Autodesk Inventor part; units mm, degrees
ref_plane "Work Plane1" through (0, 0, -16.51) normal (0, 0, 1) x (1, 0, 0)
ref_plane "Work Plane2" through (0, 0, -22.86) normal (0, 0, 1) x (1, 0, 0)
ref_plane "YZ Plane" through (0, 0, 0) normal (1, 0, 0) x (0, 1, 0)
sketch "Sketch1" plane through (0, 0, 0) normal (0, 1, 0) x (-1, 0, 0)
  line L0 (0, 0) -> (-48.9966, 0)
  line L1 (-48.9966, 0) -> (-48.9966, -45.72)
  line L2 (-48.9966, -45.72) -> (0, -45.72)
  line L3 (0, -45.72) -> (0, 0)
  dimension "d0" = 48.9966
  dimension "d1" = 45.72
extrude "Extrusion1" add sketch "Sketch1" along normal blind 6.35
sketch "Sketch3" plane through (0, 6.35, 0) normal (0, 1, 0) x (1, 0, 0)
  line L0 (0, 45.72) -> (0, 0)
  line L1 (48.9966, 0) -> (48.9966, 45.72)
  line L2 (0, 29.21) -> (48.9966, 29.21)
  line L3 (48.9966, 29.21) -> (48.9966, 16.51)
  line L4 (48.9966, 16.51) -> (0, 16.51)
  line L5 (0, 16.51) -> (0, 29.21)
  line L6 (48.9966, 45.72) -> (0, 45.72)
  dimension "d4" = 12.7
  dimension "d5" = 16.51
sketch "Sketch4" plane through (0, 6.35, 0) normal (0, 1, 0) x (1, 0, 0)
  circle A0 centre (6.35, 39.37) radius 2.1364
  circle A1 centre (42.6466, 39.37) radius 3.0733
  line L0 (48.9966, 45.72) -> (0, 45.72)
  line L1 (48.9966, 0) -> (48.9966, 45.72)
  line L2 (0, 45.72) -> (0, 0)
  circle A2 centre (6.35, 6.35) radius 2.2799
  circle A3 centre (42.6466, 6.35) radius 1.194
  line L3 (0, 0) -> (48.9966, 0)
  dimension "d6" = 6.1465
  dimension "d7" = 6.35
  dimension "d8" = 6.35
  dimension "d9" = 6.35
  dimension "d10" = 6.35
  dimension "d11" = 6.35
  dimension "d12" = 6.35
  dimension "d13" = 6.35
  dimension "d14" = 6.35
hole "Hole1" at (6.35, 6.35, -39.37) at (42.6466, 6.35, -39.37) at (42.6466, 6.35, -6.35) at (6.35, 6.35, -6.35) direction (0, -1, 0) diameter 3.4 depth 10 tip angle 118
fillet "Fillet1" radius 0.2 4 edges at (42.6466, 6.35, -41.07) (6.35, 6.35, -41.07) (42.6466, 6.35, -8.05) (6.35, 6.35, -8.05)
ref_plane "Work Plane1" through (0, 0, -16.51) normal (0, 0, 1) x (1, 0, 0)
sketch "Sketch5" plane through (0, 0, -16.51) normal (0, 0, 1) x (1, 0, 0)
  line L0 (0, 6.35) -> (48.9966, 6.35)
  line L1 (48.9966, 6.35) -> (0, 6.35)
  arc A0 (48.9966, 6.35) -> (0, 6.35) centre (24.4983, 6.35) ccw
  point P0 (0, 0)
extrude "Extrusion2" add sketch "Sketch5" along normal blind 5.08
ref_plane "Work Plane2" through (0, 0, -22.86) normal (0, 0, 1) x (1, 0, 0)
mirror "Mirror1" about plane through (0, 0, -22.86) normal (0, 0, 1) of "Extrusion2"
sketch "Sketch6" plane through (0, 0, -11.43) normal (0, 0, 1) x (1, 0, 0)
  circle A0 centre (24.4983, 17.78) radius 3.175
  line L0 (0, 6.35) -> (48.9966, 6.35)
  point P0 (0, 0)
  point P1 (24.4983, 6.35)
  point P2 (24.4983, 6.35)
  dimension "d27" = 11.43
  dimension "d28" = 6.35
extrude "Extrusion3" cut sketch "Sketch6" against normal up to surface (5.08 mm away)
sketch "Sketch8" plane through (24.4983, 6.35, -29.21) normal (0, 0, 1) x (1, 0, 0)
  circle A0 centre (0, 11.43) radius 3.175
  circle A1 centre (0, 11.43) radius 5.08
  point P0 (-24.4983, -6.35)
  dimension "d34" = 10.16
extrude "Extrusion5" cut sketch "Sketch8" against normal blind 25.4 contours A0 | A1
properties part number "Carriage Top" material "Aluminum 6061"
Here's how the part is built. I have some questions about the finished solid (model axes, mm). A direction names the side the tool comes from. Coordinates: 2 decimals unless noted, no trailing zeros. Loops run counter-clockwise (first coordinate to the right, second up) from the corner with the lowest first, then second, coordinate; pieces in that order, holes last. Notation, with made-up numbers: (64.5, 31) -> (107.5, 31) arc R23 ccw to (107.5, 53) -> close; hole circle Ø6 at (42, 21.25). An arc over 180 degrees is marked (long way). Return JSON: item names as keys, results as strings.
1) Thinking about a two-plate mould opening in Z: for faces 5 (the face through (0, 3, -23)), 6 (the face through (30, 16, -34.29)), 7 (the face through (30, 16, -29.21)), which applies, +Z half, -Z half, draft (parallel to the pull), parting line (faces both ways), or undercut?
Results below:
{"face 5": "draft", "face 6": "-Z half", "face 7": "undercut"}
2) I need wall thicknesses on line 1 (X direction, y = 1.5, z = -39.37); line 2 (Z direction, x = 6.35, y = 5.25); line 3 (Z direction, x = 6.5, y = 21.5). Which ranges of each line are inside material? Lowest first, please. Write a range as from..to.
Results below:
{"line 1": "0..4.65, 8.05..40.95, 44.35..49", "line 2": "-45.72..-41.07, -37.67..-8.05, -4.65..0", "line 3": "-34.29..-29.21, -16.51..-11.43"}
3) For faces 1 (the face through (23.837, 22.817, -31.714)), 2 (the face through (4.917, 3.032, -5.436)), 3 (the face through (25, 6.35, -6)), 4 (the face through (25, 6.35, -23)), which set-ups out of +Z, -Z, +X, -X, +Y, -Y let a thin tool reach every point of the face, with its end or its side?
Results below:
{"face 1": "-Z", "face 2": "+Y, -Y", "face 3": "+Z, +X, -X, +Y", "face 4": "+X, -X, +Y"}
4) If we section it at A-A, the plane z = -39.37: Write out the boundary of the cut face in (x, y), then the cut area to 3 significant figures.
Results below:
{"outline": "(0, 0) -> (4.65, 0) -> (4.65, 6.15) arc R0.2 ccw to (4.45, 6.35) -> (0, 6.35) -> close; (8.05, 0) -> (40.95, 0) -> (40.95, 6.15) arc R0.2 ccw to (40.75, 6.35) -> (8.25, 6.35) arc R0.2 ccw to (8.05, 6.15) -> close; (44.35, 0) -> (49, 0) -> (49, 6.35) -> (44.55, 6.35) arc R0.2 ccw to (44.35, 6.15) -> close", "area": "268 mm²"}
5) If we section it at B-B, the plane x = 6.35: Write out the boundary of the cut face in (y, z), then the cut area to 3 significant figures.
Results below:
{"outline": "(0, -45.72) -> (6.35, -45.72) -> (6.35, -41.27) arc R0.2 ccw to (6.15, -41.07) -> (0, -41.07) -> close; (0, -37.67) -> (6.15, -37.67) arc R0.2 ccw to (6.35, -37.47) -> (6.35, -34.29) -> (22.81, -34.29) -> (22.81, -29.21) -> (6.35, -29.21) -> (6.35, -16.51) -> (22.81, -16.51) -> (22.81, -11.43) -> (6.35, -11.43) -> (6.35, -8.25) arc R0.2 ccw to (6.15, -8.05) -> (0, -8.05) -> close; (0, -4.65) -> (6.15, -4.65) arc R0.2 ccw to (6.35, -4.45) -> (6.35, 0) -> (0, 0) -> close", "area": "414 mm²"}
6) If we section it at C-C, the plane y = 7: Write out the boundary of the cut face in (x, z).
Results below:
{"outline": "(0.01, -34.29) -> (48.99, -34.29) -> (48.99, -29.21) -> (0.01, -29.21) -> close; (0.01, -16.51) -> (48.99, -16.51) -> (48.99, -11.43) -> (0.01, -11.43) -> close"}
7) If we section it at D-D, the plane y = 17.78: Write out the boundary of the cut face in (x, z), then the cut area to 3 significant figures.
Results below:
{"outline": "(2.83, -34.29) -> (19.42, -34.29) -> (19.42, -29.21) -> (2.83, -29.21) -> close; (2.83, -16.51) -> (21.32, -16.51) -> (21.32, -11.43) -> (2.83, -11.43) -> close; (27.67, -16.51) -> (46.17, -16.51) -> (46.17, -11.43) -> (27.67, -11.43) -> close; (29.58, -34.29) -> (46.17, -34.29) -> (46.17, -29.21) -> (29.58, -29.21) -> close", "area": "356 mm²"}
8) Will these pins go through, and if not, where does the flat tip stop? pin 1 (7.5 mm diameter, centred on x = 18.5, y = 16, fed in from -Z); pin 2 (8 mm diameter, centred on x = 24.5, y = 17.78, fed in from -Z); pin 3 (12 mm diameter, centred on x = 35.5, y = 18.5, fed in from +Z).
Results below:
{"pin 1": "z = -34.29", "pin 2": "z = -16.51", "pin 3": "z = -11.43"}
